Print and shaded views of the part. All mm, measured from the part's lowest x, y and z. A direction names the side the tool comes from. Coordinates: 2 decimals unless noted, no trailing zeros. Order: outer loops, then holes, each group sorted by start corner. A loop starts at its lowest first (then second) coordinate and runs counter-clockwise, first axis right, second up. Notation, with made-up numbers: M 20,82 L 48,82 A30 ccw 48,113 Z; hole C 37.5,54.5 d11. An arc over 180 degrees is marked long. One line per item, written item: value.
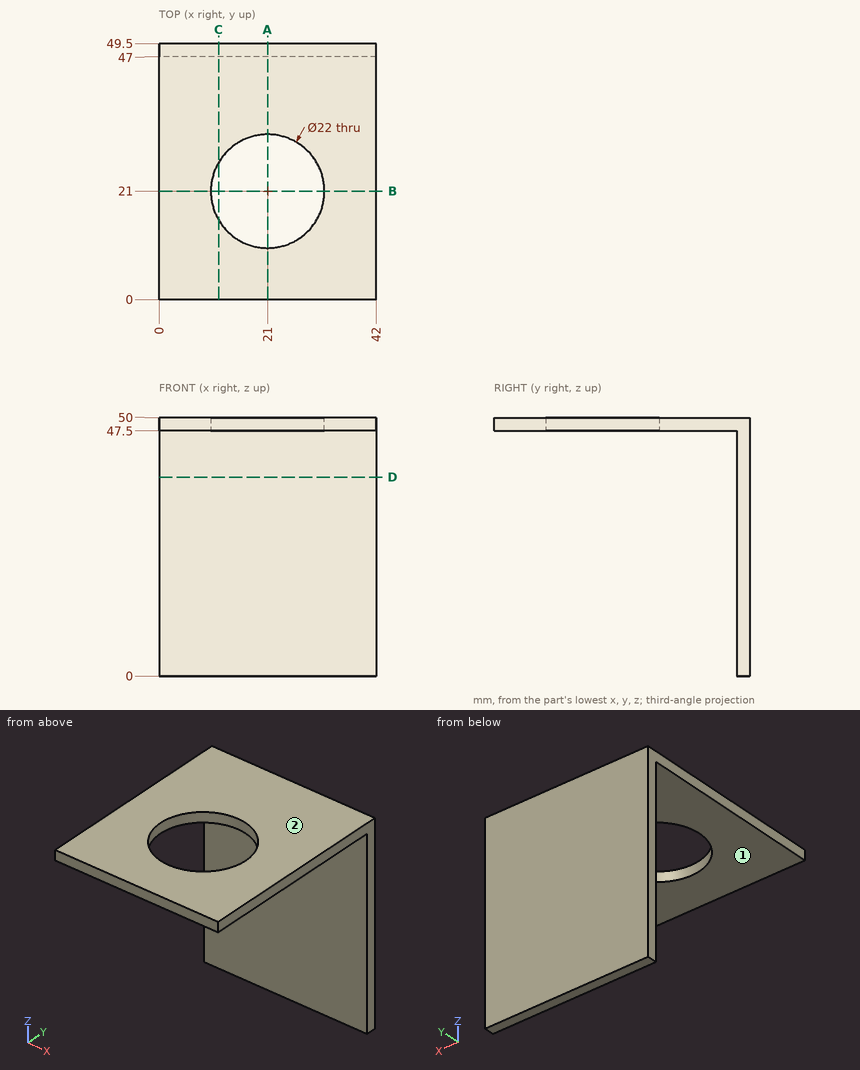
Q1. Slice it at C-C (x = 11.5). List the corners of the cut face in (y, z), plus the area to 3 significant figures.
Recorded:
outline: M 0,47.5 L 15.45,47.5 L 15.45,50 L 0,50 Z; M 26.55,47.5 L 47,47.5 L 47,0 L 49.5,0 L 49.5,50 L 26.55,50 Z
area: 215 mm^2
Q2. Pin check, flat tip, straight feed: pin 1 Ø1 at (x, y) = (37, 43.5) entering from -Z. Stop position of the tip, or through.
Recorded:
pin 1: stops at z = 47.5
Q3. Slice it at A-A (x = 21). List the corners of the cut face in (y, z), plus the area to 4 significant figures.
Recorded:
outline: M 0,47.5 L 10,47.5 L 10,50 L 0,50 Z; M 32,47.5 L 47,47.5 L 47,0 L 49.5,0 L 49.5,50 L 32,50 Z
area: 187.5 mm^2
Q4. Slice it at D-D (z = 38.5). List the corners of the cut face in (x, y).
Recorded:
outline: M 0,47 L 42,47 L 42,49.5 L 0,49.5 Z
Q5. Which spindle directions (+Z, -Z, +X, -X, +Y, -Y) get a long thin tool onto all of the face, cutting with end or side? Do the marked faces 1 and 2. Say none if no direction does.
Recorded:
face 1: -Z, +X, -X, -Y
face 2: +Z, +X, -X, +Y, -Y
Q6. Drill centre lines: line 1 along Y through (x, z) = (21, 48.4); line 2 along Y through (x, z) = (8.5, 10); line 3 along Z through (x, y) = (38.5, 33.5). Where is each one in solid material? Low to high.
Recorded:
line 1: y = 0 to 10, 32 to 49.5
line 2: y = 47 to 49.5
line 3: z = 47.5 to 50
Q7. Slice it at B-B (y = 21). List the corners of the cut face in (x, z).
Recorded:
outline: M 0,47.5 L 10,47.5 L 10,50 L 0,50 Z; M 32,47.5 L 42,47.5 L 42,50 L 32,50 Z
